Input: part model. Units: mm. Frame: model coordinates. A direction names the side the tool comes from. Coordinates: 2 decimals unless noted, no trailing zeros. Order: outer loops, then holes, each group sorted by start corner. A loop starts at its lowest first (then second) coordinate and runs counter-clockwise, first axis right, second up. Notation, with made-up numbers: (-1.75, 12) - (23.25, 12) arc R8 cw to (23.25, 16) - close; hole circle Ø8 at (-38, 86.5). An arc over 180 degrees is marked (long way). One line per question, with ' | ' between items.
Autodesk Inventor part; units mm, degrees
ref_plane "YZ Plane" through (0, 0, 0) normal (1, 0, 0) x (0, 1, 0)
ref_plane "XZ Plane" through (0, 0, 0) normal (0, 1, 0) x (-1, 0, 0)
ref_plane "XY Plane" through (0, 0, 0) normal (0, 0, 1) x (1, 0, 0)
sketch "Náčrt1" plane through (0, 0, 0) normal (1, 0, 0) x (0, 1, 0)
  line L0 (19, 6.6) -> (31.312, 6.6)
  line L1 (31.312, -6.6) -> (19, -6.6)
  line L2 (19, -6.6) -> (19, 6.6)
  line L3 (24.8085, 20.2123) -> (16.7938, 12.1976)
  line L4 (16.7938, 12.1976) -> (12.1976, 16.7938)
  line L5 (12.1976, 16.7938) -> (20.2123, 24.8085)
  line L6 (0, 0) -> (14.4957, 14.4957)
  line L7 (6.6, 19) -> (-6.6, 19)
  line L8 (6.6, 31.312) -> (6.6, 19)
  line L9 (-6.6, 19) -> (-6.6, 31.312)
  line L10 (-20.2123, 24.8085) -> (-12.1976, 16.7938)
  line L11 (-12.1976, 16.7938) -> (-16.7938, 12.1976)
  line L12 (-16.7938, 12.1976) -> (-24.8085, 20.2123)
  line L13 (-19, 6.6) -> (-19, -6.6)
  line L14 (-31.312, 6.6) -> (-19, 6.6)
  line L15 (-19, -6.6) -> (-31.312, -6.6)
  line L16 (-24.8085, -20.2123) -> (-16.7938, -12.1976)
  line L17 (-16.7938, -12.1976) -> (-12.1976, -16.7938)
  line L18 (-12.1976, -16.7938) -> (-20.2123, -24.8085)
  line L19 (-6.6, -19) -> (6.6, -19)
  line L20 (-6.6, -31.312) -> (-6.6, -19)
  line L21 (6.6, -19) -> (6.6, -31.312)
  line L22 (20.2123, -24.8085) -> (12.1976, -16.7938)
  line L23 (12.1976, -16.7938) -> (16.7938, -12.1976)
  line L24 (16.7938, -12.1976) -> (24.8085, -20.2123)
  arc A0 (24.8085, -20.2123) -> (31.312, -6.6) centre (0, 0) ccw
  arc A1 (6.6, -31.312) -> (20.2123, -24.8085) centre (0, 0) ccw
  arc A2 (-20.2123, -24.8085) -> (-6.6, -31.312) centre (0, 0) ccw
  arc A3 (-31.312, -6.6) -> (-24.8085, -20.2123) centre (0, 0) ccw
  arc A4 (-24.8085, 20.2123) -> (-31.312, 6.6) centre (0, 0) ccw
  arc A5 (-6.6, 31.312) -> (-20.2123, 24.8085) centre (0, 0) ccw
  arc A6 (31.312, 6.6) -> (24.8085, 20.2123) centre (0, 0) ccw
  arc A7 (20.2123, 24.8085) -> (6.6, 31.312) centre (0, 0) ccw
  line L25 (16.205, 20.8011) -> (20.8011, 16.205)
  line L26 (14.9675, 23.4528) -> (13.5533, 22.0386)
  line L27 (13.5533, 22.0386) -> (22.0386, 13.5533)
  line L28 (22.0386, 13.5533) -> (23.4528, 14.9675)
  line L29 (23.4528, 14.9675) -> (14.9675, 23.4528)
  line L30 (-13.5533, 22.0386) -> (-14.9675, 23.4528)
  line L31 (-22.0386, 13.5533) -> (-13.5533, 22.0386)
  line L32 (-14.9675, 23.4528) -> (-23.4528, 14.9675)
  line L33 (-23.4528, 14.9675) -> (-22.0386, 13.5533)
  line L34 (-22.0386, -13.5533) -> (-23.4528, -14.9675)
  line L35 (-13.5533, -22.0386) -> (-22.0386, -13.5533)
  line L36 (-23.4528, -14.9675) -> (-14.9675, -23.4528)
  line L37 (-14.9675, -23.4528) -> (-13.5533, -22.0386)
  line L38 (13.5533, -22.0386) -> (14.9675, -23.4528)
  line L39 (22.0386, -13.5533) -> (13.5533, -22.0386)
  line L40 (14.9675, -23.4528) -> (23.4528, -14.9675)
  line L41 (23.4528, -14.9675) -> (22.0386, -13.5533)
  point P0 (-14.4957, 14.4957)
  point P1 (-14.4957, -14.4957)
  point P2 (14.4957, -14.4957)
  dimension "d1" = 6.6
  dimension "d2" = 6.6
  dimension "d4" = 6.5
  dimension "d5" = 3.25
  dimension "d6" = 20.5
  dimension "d7" = 45
  dimension "d10" = 360
  dimension "d12" = 2
  dimension "d13" = 12
  dimension "d14" = 1
  dimension "d15" = 2.75
  dimension "d18" = 360
extrude "Vysunutí1" add sketch "Náčrt1" along normal mid plane 4 contours L2 L1 A0 L24 L40 L41 L39 L23 L22 L38 A1 L21 L19 L20 A2 L18 L36 L37 L35 L17 L16 L34 A3 L15 L13 L14 A4 L12 L32 L33 L31 L11 L10 L30 A5 L9 L7 L8 A7 L5 L29 L26 L27 L4 L3 L28 A6 L0 | L29 L28 L27 L3 | L5 L27 L26 L29 | L24 L39 L41 L40 | L40 L38 L39 L22 | L32 L30 L31 L10 | L12 L31 L33 L32 | L18 L35 L37 L36 | L36 L34 L35 L16
ref_plane "Pracovní rovina1" through (2, 0, 0) normal (1, 0, 0) x (0, 0, -1)
sketch "Náčrt2" plane through (2, 0, 0) normal (1, 0, 0) x (0, 0, -1)
  line L0 (-6.6, 19) -> (-6.6, 31.312)
  arc A0 (-6.6, 31.312) -> (-20.2123, 24.8085) centre (0, 0) ccw
  line L1 (-20.2123, 24.8085) -> (-12.1976, 16.7938)
  line L2 (-12.1976, 16.7938) -> (-16.7938, 12.1976)
  line L3 (-16.7938, 12.1976) -> (-24.8085, 20.2123)
  arc A1 (-24.8085, 20.2123) -> (-31.312, 6.6) centre (0, 0) ccw
  line L4 (-31.312, 6.6) -> (-19, 6.6)
  line L5 (-19, 6.6) -> (-19, -6.6)
  line L6 (-19, -6.6) -> (-31.312, -6.6)
  arc A2 (-31.312, -6.6) -> (-24.8085, -20.2123) centre (0, 0) ccw
  line L7 (-24.8085, -20.2123) -> (-16.7938, -12.1976)
  line L8 (-16.7938, -12.1976) -> (-12.1976, -16.7938)
  line L9 (-12.1976, -16.7938) -> (-20.2123, -24.8085)
  arc A3 (-20.2123, -24.8085) -> (-6.6, -31.312) centre (0, 0) ccw
  line L10 (-6.6, -31.312) -> (-6.6, -19)
  line L11 (-6.6, -19) -> (6.6, -19)
  line L12 (6.6, -19) -> (6.6, -31.312)
  arc A4 (6.6, -31.312) -> (20.2123, -24.8085) centre (0, 0) ccw
  line L13 (20.2123, -24.8085) -> (12.1976, -16.7938)
  line L14 (12.1976, -16.7938) -> (16.7938, -12.1976)
  line L15 (16.7938, -12.1976) -> (24.8085, -20.2123)
  arc A5 (24.8085, -20.2123) -> (31.312, -6.6) centre (0, 0) ccw
  line L16 (31.312, -6.6) -> (19, -6.6)
  line L17 (19, -6.6) -> (19, 6.6)
  line L18 (19, 6.6) -> (31.312, 6.6)
  arc A6 (31.312, 6.6) -> (24.8085, 20.2123) centre (0, 0) ccw
  line L19 (24.8085, 20.2123) -> (16.7938, 12.1976)
  line L20 (16.7938, 12.1976) -> (12.1976, 16.7938)
  line L21 (12.1976, 16.7938) -> (20.2123, 24.8085)
  arc A7 (20.2123, 24.8085) -> (6.6, 31.312) centre (0, 0) ccw
  line L22 (6.6, 31.312) -> (6.6, 19)
  line L23 (6.6, 19) -> (-6.6, 19)
  line L24 (-16.7938, 12.1976) -> (-24.8085, 20.2123)
  line L25 (-20.8011, 16.205) -> (-16.205, 20.8011)
  line L26 (-23.4528, 14.9675) -> (-14.9675, 23.4528)
  line L27 (-20.2123, 24.8085) -> (-12.1976, 16.7938)
  line L28 (-14.9675, 23.4528) -> (-13.5533, 22.0386)
  line L29 (-13.5533, 22.0386) -> (-22.0386, 13.5533)
  line L30 (-22.0386, 13.5533) -> (-23.4528, 14.9675)
  line L31 (-16.205, -20.8011) -> (-20.8011, -16.205)
  line L32 (-22.0386, -13.5533) -> (-13.5533, -22.0386)
  line L33 (-14.9675, -23.4528) -> (-23.4528, -14.9675)
  line L34 (-13.5533, -22.0386) -> (-14.9675, -23.4528)
  line L35 (-23.4528, -14.9675) -> (-22.0386, -13.5533)
  line L36 (20.8011, -16.205) -> (16.205, -20.8011)
  line L37 (13.5533, -22.0386) -> (22.0386, -13.5533)
  line L38 (23.4528, -14.9675) -> (14.9675, -23.4528)
  line L39 (22.0386, -13.5533) -> (23.4528, -14.9675)
  line L40 (14.9675, -23.4528) -> (13.5533, -22.0386)
  line L41 (16.205, 20.8011) -> (20.8011, 16.205)
  line L42 (22.0386, 13.5533) -> (13.5533, 22.0386)
  line L43 (14.9675, 23.4528) -> (23.4528, 14.9675)
  line L44 (13.5533, 22.0386) -> (14.9675, 23.4528)
  line L45 (23.4528, 14.9675) -> (22.0386, 13.5533)
  dimension "d23" = 12
  dimension "d24" = 2
  dimension "d25" = 1
  dimension "d26" = 2.75
  dimension "d27" = 6.5
  dimension "d30" = 360
extrude "Vysunutí2" cut sketch "Náčrt2" against normal blind 2.5 contours L26 L28 L29 L1 | L1 L25 L3 L26 | L1 L29 L3 L25 | L3 L29 L30 L26 | L43 L19 L41 L21 | L21 L42 L44 L43 | L41 L19 L42 L21 | L43 L45 L42 L19 | L33 L35 L32 L7 | L7 L31 L9 L33 | L7 L32 L9 L31 | L9 L32 L34 L33 | L38 L13 L36 L15 | L15 L37 L39 L38 | L36 L13 L37 L15 | L38 L40 L37 L13
sketch "Náčrt3" plane through (2, 0, 0) normal (1, 0, 0) x (0, 0, -1)
  line L0 (-11.5, 7) -> (-11.5, -7)
  line L1 (11.5, -7) -> (11.5, 7)
  arc A0 (5, 7) -> (-5, 7) centre (0, 7) ccw
  arc A1 (-5, -7) -> (5, -7) centre (0, -7) ccw
  line L2 (-11.5, -7) -> (-5, -7)
  line L3 (5, -7) -> (11.5, -7)
  line L4 (11.5, 7) -> (5, 7)
  line L5 (-5, 7) -> (-11.5, 7)
  point P0 (0, 0)
  dimension "d34" = 23
  dimension "d35" = 14
  dimension "d37" = 11.5
  dimension "d38" = 10
  dimension "d39" = 10
extrude "Vysunutí3" cut sketch "Náčrt3" against normal blind 4
ref_plane "Pracovní rovina2" through (-2, 0, 0) normal (-1, 0, 0) x (0, 0, 1)
sketch "Náčrt4" plane through (-2, 0, 0) normal (-1, 0, 0) x (0, 0, 1)
  line L0 (-11.5, 7) -> (-5, 7)
  arc A0 (5, 7) -> (-5, 7) centre (0, 7) ccw
  line L1 (5, 7) -> (11.5, 7)
  line L2 (11.5, 7) -> (11.5, -7)
  line L3 (11.5, -7) -> (5, -7)
  arc A1 (-5, -7) -> (5, -7) centre (0, -7) ccw
  line L4 (-5, -7) -> (-11.5, -7)
  line L5 (-11.5, -7) -> (-11.5, 7)
  line L6 (6.6, 31.312) -> (6.6, 19)
  line L7 (6.6, 19) -> (-6.6, 19)
  line L8 (-6.6, 19) -> (-6.6, 31.312)
  arc A2 (-6.6, 31.312) -> (-20.2123, 24.8085) centre (0, 0) ccw
  line L9 (-20.2123, 24.8085) -> (-12.1976, 16.7938)
  line L10 (-12.1976, 16.7938) -> (-16.7938, 12.1976)
  line L11 (-16.7938, 12.1976) -> (-24.8085, 20.2123)
  arc A3 (-24.8085, 20.2123) -> (-31.312, 6.6) centre (0, 0) ccw
  line L12 (-31.312, 6.6) -> (-19, 6.6)
  line L13 (-19, 6.6) -> (-19, -6.6)
  line L14 (-19, -6.6) -> (-31.312, -6.6)
  arc A4 (-31.312, -6.6) -> (-24.8085, -20.2123) centre (0, 0) ccw
  line L15 (-24.8085, -20.2123) -> (-16.7938, -12.1976)
  line L16 (-16.7938, -12.1976) -> (-12.1976, -16.7938)
  line L17 (-12.1976, -16.7938) -> (-20.2123, -24.8085)
  arc A5 (-20.2123, -24.8085) -> (-6.6, -31.312) centre (0, 0) ccw
  line L18 (-6.6, -31.312) -> (-6.6, -19)
  line L19 (-6.6, -19) -> (6.6, -19)
  line L20 (6.6, -19) -> (6.6, -31.312)
  arc A6 (6.6, -31.312) -> (20.2123, -24.8085) centre (0, 0) ccw
  line L21 (20.2123, -24.8085) -> (12.1976, -16.7938)
  line L22 (12.1976, -16.7938) -> (16.7938, -12.1976)
  line L23 (16.7938, -12.1976) -> (24.8085, -20.2123)
  arc A7 (24.8085, -20.2123) -> (31.312, -6.6) centre (0, 0) ccw
  line L24 (31.312, -6.6) -> (19, -6.6)
  line L25 (19, -6.6) -> (19, 6.6)
  line L26 (19, 6.6) -> (31.312, 6.6)
  arc A8 (31.312, 6.6) -> (24.8085, 20.2123) centre (0, 0) ccw
  line L27 (24.8085, 20.2123) -> (16.7938, 12.1976)
  line L28 (16.7938, 12.1976) -> (12.1976, 16.7938)
  line L29 (12.1976, 16.7938) -> (20.2123, 24.8085)
  arc A9 (20.2123, 24.8085) -> (6.6, 31.312) centre (0, 0) ccw
  line L30 (16.7938, 12.1976) -> (12.1976, 16.7938)
  line L31 (-16.7938, -12.1976) -> (-12.1976, -16.7938)
sketch "Náčrt5" plane through (-2, 0, 0) normal (-1, 0, 0) x (0, 0, 1)
  circle A0 centre (10, -10) radius 1.5
  circle A1 centre (10, 10) radius 1.5
  circle A2 centre (-10, 10) radius 1.5
  circle A3 centre (-10, -10) radius 1.5
  point P0 (0, 0)
  dimension "d45" = 360
  dimension "d47" = 10
  dimension "d48" = 10
  dimension "d49" = 3
extrude "Vysunutí4" cut sketch "Náčrt5" against normal blind 4
sketch "Náčrt6" plane through (2, 0, 0) normal (1, 0, 0) x (0, 0, -1)
  circle A0 centre (10, 25) radius 1.25
  circle A1 centre (-10, 25) radius 1.25
  circle A2 centre (-25, 10) radius 1.25
  circle A3 centre (-25, -10) radius 1.25
  circle A4 centre (-10, -25) radius 1.25
  circle A5 centre (10, -25) radius 1.25
  circle A6 centre (25, -10) radius 1.25
  circle A7 centre (25, 10) radius 1.25
  point P0 (0, 0)
  dimension "d52" = 2.5
  dimension "d53" = 2.5
  dimension "d54" = 25
  dimension "d55" = 25
  dimension "d56" = 10
  dimension "d57" = 10
  dimension "d60" = 360
extrude "Vysunutí5" cut sketch "Náčrt6" against normal blind 4
equation "\"d5\" = 0.5 * d4"
equation "\"d14\" = 0.5 * d12"
equation "\"d15\" = -0.5 * d4 + 0.5 * d13"
equation "\"d25\" = 0.5 * d24"
equation "\"d26\" = -0.5 * d27 + 0.5 * d23"
equation "\"d39\" = d38"
equation "\"d53\" = d52"
equation "\"d36\" = 0.5 * d35"
properties part number "deska"
Item 1: Section B-B on z = -10. Return the cut outline in (x, y), and give its area (3 significant figures).
Data:
outline: (-2, -30.4) - (2, -30.4) - (2, -26.25) - (-2, -26.25) - close; (-2, -23.75) - (2, -23.75) - (2, -11.5) - (-2, -11.5) - close; (-2, -8.5) - (2, -8.5) - (2, -7) - (-2, -7) - close; (-2, 7) - (2, 7) - (2, 8.5) - (-2, 8.5) - close; (-2, 11.5) - (2, 11.5) - (2, 23.75) - (-2, 23.75) - close; (-2, 26.25) - (2, 26.25) - (2, 30.4) - (-2, 30.4) - close | area: 143 mm^2
Item 2: Section A-A on y = -2. Return the cut outline in (x, z).
Data:
outline: (-2, -19) - (2, -19) - (2, -11.5) - (-2, -11.5) - close; (-2, 11.5) - (2, 11.5) - (2, 19) - (-2, 19) - close
Item 3: Section D-D on y = 10. Return the cut outline in (x, z).
Data:
outline: (-2, -30.4) - (2, -30.4) - (2, -26.25) - (-2, -26.25) - close; (-2, -23.75) - (2, -23.75) - (2, -11.5) - (-2, -11.5) - close; (-2, -8.5) - (2, -8.5) - (2, -4) - (-2, -4) - close; (-2, 4) - (2, 4) - (2, 8.5) - (-2, 8.5) - close; (-2, 11.5) - (2, 11.5) - (2, 23.75) - (-2, 23.75) - close; (-2, 26.25) - (2, 26.25) - (2, 30.4) - (-2, 30.4) - close
Item 4: Contact query for flat-ended pins moving along their axis: P1, Ø2.5, axis at y = 10, z = 10, coming from the +X side; P2, Ø1.2, axis at x = -0.5, y = 1, coming from the +Z side; P3, Ø1.5, axis at x = 0.5, y = 16, coming from the -Z side; P4, Ø1, axis at y = 16, z = 21.5, coming from the +X side. Output: stop coordinate, or through.
Data:
P1: through | P2: z = 19 | P3: z = -28.13 | P4: x = -0.5
Item 5: Section C-C on x = -1.3. Count the separate pieces of the cut face and the enclosed holes in it, and give its area (3 significant figures).
Data:
separate pieces: 1 | enclosed holes: 13 | area: 1,780 mm^2
Item 6: Draft query along Y for faces 4 (the face through (0, 25, 6.6)), 5 (the face through (0, 7, -8)), 6 (the face through (-0.03, 28.92, -13.7)), 7 (the face through (0, 9.1, -11.2)). Return one class per face: released by +Y, released by -Y, zero draft, split by the parting line, or undercut.
Data:
face 4: zero draft | face 5: undercut | face 6: released by +Y | face 7: undercut
Item 7: Access query for faces 1 (the face through (0, 0, -19)), 2 (the face through (0.77, -22.49, 15.93)), 3 (the face through (-0.917, 20.745, -16.149)). Directions: +Z, -Z, +X, -X, +Y, -Y. A direction counts if a zero-diameter tool reaches every point of the face in a straight line with its end or side. Return the directions, or none.
Data:
face 1: -Z, +X, -X | face 2: +X | face 3: +X, -X
Item 8: Ray query, line 1 (Z direction, x = 1.35, y = 4); line 2 (Z direction, x = 0.65, y = 14); line 3 (Z direction, x = -1.1, y = -15). Return the intervals inside material, ascending.
Data:
line 1: -19 to -11.5, 11.5 to 19 | line 2: -28.78 to -22.49, -21.59 to -18.6, -14.99 to 14.99, 18.6 to 21.59, 22.49 to 28.77 | line 3: -28.27 to -19.6, -13.99 to 13.99, 19.6 to 28.27
